Build history of the part. All positions in model axes, mm. A direction names the side the tool comes from. Round coordinates to 2 decimals unless told otherwise and drop trailing zeros. Order: outer loops, then holes, each group sorted by start corner. A loop starts at its lowest first (then second) coordinate and runs counter-clockwise, first axis right, second up. Notation, with made-up numbers: (-1.5, -10) - (54.5, -10) arc R31 ccw to (54.5, 18) - close; hole circle Ø8 at (65, 6.25). An arc over 180 degrees is marked (long way). Write each question's results on one line, items separated by ' | '. Start each with the question number.
```python
from build123d import *

# Parameters (mm, degrees)
SKETCH1_R           = 2.5
BOSS_EXTRUDE1_DEPTH = 46.04
SKETCH3_W           = 18.51
SKETCH3_H           = 3
CUT_EXTRUDE1_DEPTH  = 0.5
CHAMFER1_SIZE       = 0.5


with BuildPart() as part:
    # Sketch1 → Boss-Extrude1 (new body)
    with BuildSketch(Plane(origin=(0, 0, 0), x_dir=(0, 0, -1), z_dir=(1, 0, 0))):
        Circle(SKETCH1_R)
    extrude(amount=BOSS_EXTRUDE1_DEPTH)

    # Sketch3 → Cut-Extrude1 (cut)
    with BuildSketch(Plane(origin=(0, 2.5, 0), x_dir=(1, 0, 0), z_dir=(0, 1, 0))):
        with Locations((36.785, 0)):
            Rectangle(SKETCH3_W, SKETCH3_H)
    extrude(amount=-CUT_EXTRUDE1_DEPTH, mode=Mode.SUBTRACT)

    # Chamfer1
    chamfer1_edges = [part.edges().sort_by_distance(p)[0] for p in [
        (46.04, -2.236067977, 1.118033989),
        (46.04, 2, 0),
    ]]
    chamfer(chamfer1_edges, length=CHAMFER1_SIZE - 0.0001)  # a hair under: the kernel refuses the full size


solid = part.part
```
1. Cut at B-B (x = 7.5). List the corners of the cut face in (y, z), plus the area to 3 significant figures.
2. Wall check: line 1 (Z direction, x = 3.5, y = -0.15); line 2 (Z direction, x = 16, y = 1.5); line 3 (Y direction, x = 18.5, z = 0.2). Give the ranges that are in metal, low to high. Write a range as from..to.
3. 3-axis set-ups, long thin cutter, end or side, ignore diameter. For faces 1 (the face through (36, 2, 0)), 2 (the face through (45.905, -2.134, 0.075)): which of +Z, -Z, +X, -X, +Y, -Y reach the whole face in a straight line?
4. Flat gauge pin, fed straight in: pin 1 Ø1 at (x, z) = (7, 1.5) entering from -Y. Where does the tip first touch, or does it go through?
5. Cut at A-A (z = 0). List the corners of the cut face in (x, y), plus the area to 3 significant figures.
A:
1) outline: circle Ø5 at (0, 0) | area: 19.6 mm^2
2) line 1: z = -2.5..2.5 | line 2: z = -2..2 | line 3: y = -2.49..2.49
3) face 1: +Z, -Z, +X, +Y | face 2: +X
4) pin 1: stops at y = -2.29
5) outline: (0, -2.5) - (45.54, -2.5) - (46.04, -2) - (46.04, 1.5) - (45.54, 2) - (27.53, 2) - (27.53, 2.5) - (0, 2.5) - close | area: 221 mm^2
